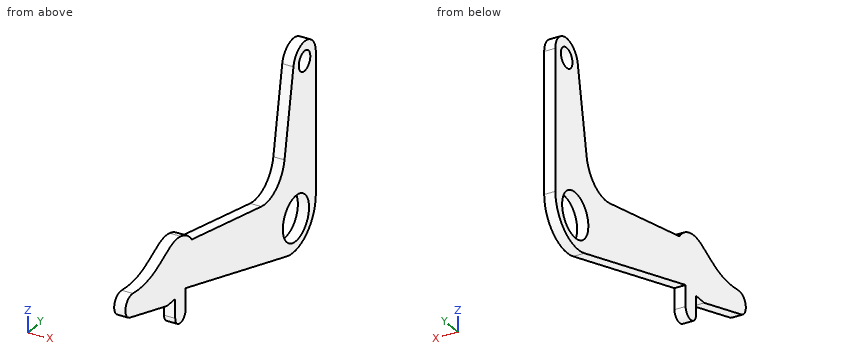
from build123d import *

# Parameters (mm, degrees)
SKETCH1_R           = 5.1308
SKETCH1_R_2         = 2.262010882
BOSS_EXTRUDE1_DEPTH = 2.54


with BuildPart() as part:
    # Sketch1 → Boss-Extrude1 (new body)
    with BuildSketch(Plane(origin=(0, 0, 0), x_dir=(0, 0, -1), z_dir=(1, 0, 0))):
        with BuildLine():
            Line((-32.256192364, 8.796557636), (0, 8.796557636))
            ThreePointArc((0, 8.796557636), (7.072772121, 5.230231425), (8.410616185, -2.577006332))
            Line((8.410616185, -2.577006332), (-3.731873822, -42.206642364))
            Line((-3.731873822, -42.206642364), (1.115138458, -42.206642364))
            ThreePointArc((1.115138458, -42.206642364), (3.134438458, -44.225942364), (1.115138458, -46.245242364))
            Line((1.115138458, -46.245242364), (-3.266361542, -46.245242364))
            Line((-3.266361542, -46.245242364), (-3.266361542, -49.521842364))
            Line((-3.266361542, -49.521842364), (-7.701250082, -63.996057998))
            ThreePointArc((-7.701250082, -63.996057998), (-10.694320166, -65.70408502), (-12.581554006, -62.820654204))
            add(Edge.make_bspline(
                [(-16.349353221, -44.121567363), (-17.528227781, -49.64987319), (-11.082221769, -52.675290574), (-12.581554006, -62.820654204)],
                knots=[0, 0, 0, 0, 1, 1, 1, 1], degree=3))
            ThreePointArc((-16.349353221, -44.121567363), (-15.336629179, -41.682166261), (-13.516414071, -39.768242364))
            Line((-13.516414071, -39.768242364), (-7.67265893, -12.543758648))
            ThreePointArc((-7.67265893, -12.543758648), (-8.792024721, -6.703826274), (-13.766553539, -3.446242364))
            Line((-13.766553539, -3.446242364), (-33.041775294, 0.040539507))
            ThreePointArc((-33.041775294, 0.040539507), (-36.651786579, 4.777676826), (-32.256192364, 8.796557636))
        make_face()
        with Locations((1.580189797, 1.024157636)):
            Circle(SKETCH1_R, mode=Mode.SUBTRACT)
        with Locations((-32.256192364, 4.383307636)):
            Circle(SKETCH1_R_2, mode=Mode.SUBTRACT)
    extrude(amount=BOSS_EXTRUDE1_DEPTH)


solid = part.part
Model file for the job. Use its own axes, mm. Give positions to 0.01 mm unless a question says otherwise; leave off trailing zeros. Order: outer loops, then holes, each group sorted by start corner. A loop starts at its lowest first (then second) coordinate and runs counter-clockwise, first axis right, second up. Notation, with made-up numbers: (37, 24) - (72, 24) arc R29 ccw to (72, 61) - close; hole circle Ø11 at (62.5, 83). An arc over 180 degrees is marked (long way). Write item = value, one per line. Start each with the question number.
1. Drop flat-ended pins along their axis: P1, Ø0.8, axis at x = 1.5, z = 2, coming from the -Y side; P2, Ø16.5, axis at y = 1.02, z = -1.58, coming from the -X side. Give the stop position or say it passes through.
2. Cut at B-B, the plane z = 11. List the corners of the cut face in (x, y).
3. Cut at D-D, the plane y = -30.5. List the corners of the cut face in (x, z).
4. Cut at A-A, the plane z = -2. List the corners of the cut face in (x, y), and give its area (3 significant figures).
5. Probe line 1 along Z through (x, y) = (2.2, 4); line 2 along Z through (x, y) = (0.85, 4.5); line 3 along Y through (x, z) = (2.2, 34). List the from-to ranges inside material, lowest first.
6. Cut at C-C, the plane x = 0.6. State how many separate pieces and enclosed holes the cut face has, and give its area (3 significant figures).
Taken from the geometry:
q1.P1 = -46.25
q1.P2 = 0
q2.outline = (0, -65.61) - (2.54, -65.61) - (2.54, -28.04) - (0, -28.04) - close; (0, -4.54) - (2.54, -4.54) - (2.54, 8.8) - (0, 8.8) - close
q3.outline = (0, 0.14) - (2.54, 0.14) - (2.54, 11.53) - (0, 11.53) - close
q4.outline = (0, -46.04) - (2.54, -46.04) - (2.54, -42.41) - (0, -42.41) - close; (0, -23.5) - (2.54, -23.5) - (2.54, -4.09) - (0, -4.09) - close; (0, 6.14) - (2.54, 6.14) - (2.54, 8.57) - (0, 8.57) - close
q4.area = 64.7 mm²
q5.line_1 = -7.83 to -5.76, 2.6 to 30.03, 34.49 to 36.65
q5.line_2 = -7.56 to -5.35, 2.19 to 30, 34.52 to 36.67
q5.line_3 = 0.33 to 2.94, 5.82 to 8.44
q6.separate_pieces = 1
q6.enclosed_holes = 2
q6.area = 1,110 mm²
